```python
from build123d import *

# Parameters (mm, degrees)
SKIZZE1_W                       = 450
SKIZZE1_H                       = 310
AUFSATZ_LINEAR_AUSTRAGEN1_DEPTH = 5
SKIZZE2_W                       = 10
SKIZZE2_H                       = 10
SKIZZE2_W_2                     = 25
SCHNITT_LINEAR_AUSTRAGEN1_DEPTH = 547.465918425
SKIZZE3_W                       = 5
SKIZZE3_H                       = 100
SCHNITT_LINEAR_AUSTRAGEN2_DEPTH = 547.465918425
SKIZZE4_W                       = 20
SKIZZE4_H                       = 5
SCHNITT_LINEAR_AUSTRAGEN3_DEPTH = 547.465918425
SKIZZE5_R                       = 1.5
SCHNITT_LINEAR_AUSTRAGEN4_DEPTH = 547.465918425
SKIZZE6_R                       = 2
SCHNITT_LINEAR_AUSTRAGEN5_DEPTH = 547.465918425


with BuildPart() as part:
    # Skizze1 → Aufsatz-Linear austragen1 (new body)
    with BuildSketch(Plane(origin=(0, 0, 0), x_dir=(1, 0, 0), z_dir=(0, 1, 0))):
        with Locations((225, -155)):
            Rectangle(SKIZZE1_W, SKIZZE1_H)
    extrude(amount=AUFSATZ_LINEAR_AUSTRAGEN1_DEPTH)

    # Skizze2 → Schnitt-Linear austragen1 (cut, through all)
    with BuildSketch(Plane(origin=(0, 5, 0), x_dir=(1, 0, 0), z_dir=(0, 1, 0))):
        with Locations((5, -5)):
            Rectangle(SKIZZE2_W, SKIZZE2_H)
        with Locations((445, -305)):
            Rectangle(SKIZZE2_W, SKIZZE2_H)
        with Locations((445, -5)):
            Rectangle(SKIZZE2_W, SKIZZE2_H)
        with Locations((5, -305)):
            Rectangle(SKIZZE2_W, SKIZZE2_H)
        with Locations((82.5, -5)):
            Rectangle(SKIZZE2_W_2, SKIZZE2_H)
        with Locations((327.5, -5)):
            Rectangle(SKIZZE2_W_2, SKIZZE2_H)
        with Locations((327.5, -305)):
            Rectangle(SKIZZE2_W_2, SKIZZE2_H)
        with Locations((82.5, -305)):
            Rectangle(SKIZZE2_W_2, SKIZZE2_H)
    extrude(amount=-SCHNITT_LINEAR_AUSTRAGEN1_DEPTH, mode=Mode.SUBTRACT)

    # Skizze3 → Schnitt-Linear austragen2 (cut, through all)
    with BuildSketch(Plane(origin=(0, 5, 0), x_dir=(1, 0, 0), z_dir=(0, 1, 0))):
        with Locations((82.5, -155)):
            Rectangle(SKIZZE3_W, SKIZZE3_H)
        with Locations((327.5, -155)):
            Rectangle(SKIZZE3_W, SKIZZE3_H)
    extrude(amount=-SCHNITT_LINEAR_AUSTRAGEN2_DEPTH, mode=Mode.SUBTRACT)

    # Skizze4 → Schnitt-Linear austragen3 (cut, through all)
    with BuildSketch(Plane(origin=(0, 5, 0), x_dir=(1, 0, 0), z_dir=(0, 1, 0))):
        with Locations((115, -287.5)):
            Rectangle(SKIZZE4_W, SKIZZE4_H)
        with Locations((295, -287.5)):
            Rectangle(SKIZZE4_W, SKIZZE4_H)
        with Locations((115, -237.5)):
            Rectangle(SKIZZE4_W, SKIZZE4_H)
        with Locations((115, -187.5)):
            Rectangle(SKIZZE4_W, SKIZZE4_H)
        with Locations((115, -137.5)):
            Rectangle(SKIZZE4_W, SKIZZE4_H)
        with Locations((115, -87.5)):
            Rectangle(SKIZZE4_W, SKIZZE4_H)
        with Locations((295, -237.5)):
            Rectangle(SKIZZE4_W, SKIZZE4_H)
        with Locations((295, -187.5)):
            Rectangle(SKIZZE4_W, SKIZZE4_H)
        with Locations((295, -137.5)):
            Rectangle(SKIZZE4_W, SKIZZE4_H)
        with Locations((295, -87.5)):
            Rectangle(SKIZZE4_W, SKIZZE4_H)
    extrude(amount=-SCHNITT_LINEAR_AUSTRAGEN3_DEPTH, mode=Mode.SUBTRACT)

    # Skizze5 → Schnitt-Linear austragen4 (cut, through all)
    with BuildSketch(Plane(origin=(0, 5, 0), x_dir=(1, 0, 0), z_dir=(0, 1, 0))):
        with Locations(Location((40, -10, 0), (0, 0, 270))):
            Circle(SKIZZE5_R)
        with Locations(Location((205, -10, 0), (0, 0, 270))):
            Circle(SKIZZE5_R)
        with Locations(Location((390, -10, 0), (0, 0, 270))):
            Circle(SKIZZE5_R)
        with Locations(Location((40, -300, 0), (0, 0, 270))):
            Circle(SKIZZE5_R)
        with Locations(Location((205, -300, 0), (0, 0, 270))):
            Circle(SKIZZE5_R)
        with Locations(Location((390, -300, 0), (0, 0, 270))):
            Circle(SKIZZE5_R)
    extrude(amount=-SCHNITT_LINEAR_AUSTRAGEN4_DEPTH, mode=Mode.SUBTRACT)

    # Skizze6 → Schnitt-Linear austragen5 (cut, through all)
    with BuildSketch(Plane(origin=(0, 5, 0), x_dir=(1, 0, 0), z_dir=(0, 1, 0))):
        with Locations(Location((40, -270, 0), (0, 0, 270))):
            Circle(SKIZZE6_R)
    extrude(amount=-SCHNITT_LINEAR_AUSTRAGEN5_DEPTH, mode=Mode.SUBTRACT)


solid = part.part
```
Check sheet for the modelled part. Datum: model origin and axes. Units: mm. Coordinates: 2 decimals unless noted, no trailing zeros. Write item = value, one per line. Start each with the question number.
1. Thickness scan on probe 1 along X at (y, z) = (4.65, 132); probe 2 along Z at (x, y) = (292, 1.75); probe 3 along Z at (x, y) = (205, 1.25). Record the ranges inside material, lowest first.
2. Go/stop test with flat-tipped pins: pin 1 (2.5 mm diameter, centred on y = 1.5, z = 303, fed in from +X); pin 2 (2.5 mm diameter, centred on x = 330, y = 3.5, fed in from -Z). Record where each tip stops, or that it passes through.
3. Sectioned sample at A-A (y = 0.8). State how many separate pieces and enclosed holes the cut face has, then the cut area to 3 significant figures.
The answers:
q1.probe_1 = 0 to 80, 85 to 325, 330 to 450
q1.probe_2 = 0 to 85, 90 to 135, 140 to 185, 190 to 235, 240 to 285, 290 to 310
q1.probe_3 = 0 to 8.5, 11.5 to 298.5, 301.5 to 310
q2.pin_1 = 440
q2.pin_2 = 10
q3.separate_pieces = 1
q3.enclosed_holes = 19
q3.area = 136,000 mm²
